Verification items for the finished model (mm, model axes). A direction names the side the tool comes from. Round coordinates to 2 decimals unless told otherwise and drop trailing zeros. Write each loop counter-clockwise with the first axis right and the second up, starting at its lowest first coordinate (ties: lowest second). Pieces come first, ordered by that corner, then holes. Notation, with made-up numbers: M 57,-26 L 76,-26 A23 ccw 76,0 Z; hole C -3.5,-6 d11. An arc over 180 degrees is marked long. One line per item, written item: value. Start each with the question number.
Item 1: Section check A-A, the plane x = -42. Record the cut outline in (y, z), then the cut area to 3 significant figures.
Item 2: Section check B-B, the plane y = -36. Record the cut outline in (x, z), then the cut area to 3 significant figures.
Item 3: Gauge pin test, flat ends, axial feed: pin 1 (14.5 mm diameter, centred on y = 8.5, z = 62.5, fed in from +X); pin 2 (12 mm diameter, centred on y = -6.5, z = 33, fed in from +X); pin 3 (23 mm diameter, centred on x = 38, z = 7.5, fed in from -Y). Record the tip position at first contact, or that the pin passes through.
Item 4: Draft check along X on faces 4 (the face through (-30, 1, 25.4)), 5 (the face through (53.34, 0, 13)), 6 (the face through (-5.74, 28, 13)), 7 (the face through (1.12, -16.22, 12.2)). Enter one of: +X half, -X half, draft (parallel to the pull), parting line (faces both ways), or undercut.
Item 5: Section check C-C, the plane z = 6. Record the cut outline in (x, y).
Item 6: Tool access check on faces 1 (the face through (8.557, 27, 13)), 2 (the face through (1, -22, 24.745)), 3 (the face through (38, -31.519, 13)). Record the directions out of +Z, -Z, +X, -X, +Y, -Y that give a thin tool (end or side, any length) a straight path to the whole face; none if there is none.
Item 7: Thickness scan on probe 1 along Y at (x, z) = (-44, 10); probe 2 along X at (y, z) = (22, 20.5); probe 3 along X at (y, z) = (0, 64). Record the ranges inside material, lowest first. Write a range as from..to.
from build123d import *

# Parameters (mm, degrees)
F1_DEPTH       = 25.4
F2_R           = 5.4495134178
F2_R_2         = 5.5089125438
F3_DEPTH       = 25.4
F4_R           = 5.1025387704
F4_R_2         = 4.874193153
F5_DEPTH       = 25.4
F7_DEPTH       = 25.4
F9_DEPTH       = 25.4
F10_R          = 5.08
F15_R          = 7.7344411216
F16_DEPTH      = 25.4
F17_W          = 15.24
F17_H          = 33.801519665
F18_DEPTH      = 25.4
F18_DEPTH_BACK = 25.4


# Not quite as in the source:
# - a feature of the source that left no trace in its solid (it failed there, or was rolled back) is left out


with BuildPart() as f1:
    # F0 (on Top) → F1 (new body)
    with BuildSketch(Plane.XY):
        with BuildLine():
            Line((-53.3399991691, -31.5190926194), (-27.1817994649, -31.5190926194))
            ThreePointArc((-27.1817994649, -31.5190926194), (-41.6209493128, 0), (-27.1817994649, 31.5190926194))
            Line((-27.1817994649, 31.5190926194), (-53.3399991691, 31.5190926194))
            Line((-53.3399991691, 31.5190926194), (-53.3399991691, -31.5190926194))
        make_face()
        with BuildLine():
            Line((27.1817994649, -31.5190926194), (53.3399991691, -31.5190926194))
            Line((53.3399991691, -31.5190926194), (53.3399991691, 31.5190926194))
            Line((53.3399991691, 31.5190926194), (27.1817994649, 31.5190926194))
            ThreePointArc((27.1817994649, 31.5190926194), (37.8393691772, 17.3345193752), (41.6209493128, 0))
            ThreePointArc((41.6209493128, 0), (37.8393691772, -17.3345193752), (27.1817994649, -31.5190926194))
        make_face()
        with BuildLine():
            ThreePointArc((-27.1817994649, -31.5190926194), (0, -41.6209493128), (27.1817994649, -31.5190926194))
            Line((27.1817994649, -31.5190926194), (-27.1817994649, -31.5190926194))
        make_face()
        with BuildLine():
            Line((-27.1817994649, 31.5190926194), (27.1817994649, 31.5190926194))
            ThreePointArc((27.1817994649, 31.5190926194), (0, 41.6209493128), (-27.1817994649, 31.5190926194))
        make_face()
        with BuildLine():
            Line((-27.1817994649, -31.5190926194), (27.1817994649, -31.5190926194))
            ThreePointArc((27.1817994649, -31.5190926194), (37.8393691772, -17.3345193752), (41.6209493128, 0))
            ThreePointArc((41.6209493128, 0), (37.8393691772, 17.3345193752), (27.1817994649, 31.5190926194))
            Line((27.1817994649, 31.5190926194), (-27.1817994649, 31.5190926194))
            ThreePointArc((-27.1817994649, 31.5190926194), (-41.6209493128, 0), (-27.1817994649, -31.5190926194))
        make_face()
    extrude(amount=F1_DEPTH)

    # F2 (on face) → F3 (cut)
    with BuildSketch(Plane.XY.offset(25.4)):
        with Locations((-44.2123003304, 23.8175932318)):
            Circle(F2_R)
        with Locations((-43.9270585775, -22.6766318083)):
            Circle(F2_R_2)
    extrude(amount=-F3_DEPTH, mode=Mode.SUBTRACT)

    # F4 (on face) → F5 (cut)
    with BuildSketch(Plane.XY.offset(25.4)):
        with Locations((46.7794649303, 24.6733147651)):
            Circle(F4_R)
        with Locations((46.2089851499, -25.2437964082)):
            Circle(F4_R_2)
    extrude(amount=-F5_DEPTH, mode=Mode.SUBTRACT)

    # F6 (on face) → F7 (cut)
    with BuildSketch(Plane.XY.offset(25.4)):
        with BuildLine():
            Line((-6.9852194627, -11.5522462875), (-6.9852194627, -41.0305999317))
            Line((-6.9852194627, -41.0305999317), (6.9852194627, -41.0305999317))
            ThreePointArc((6.9852194627, -41.0305999317), (8.0592339465, -40.8332238489), (9.1277007014, -40.6077394299))
            Line((9.1277007014, -40.6077394299), (9.1277007014, -11.5522462875))
            Line((9.1277007014, -11.5522462875), (-6.9852194627, -11.5522462875))
        make_face()
        with BuildLine():
            Line((6.9852194627, -41.0305999317), (-6.9852194627, -41.0305999317))
            ThreePointArc((-6.9852194627, -41.0305999317), (0, -41.6209493128), (6.9852194627, -41.0305999317))
        make_face()
        with BuildLine():
            Line((5.7398033244, 41.2232710917), (-5.7398033244, 41.2232710917))
            Line((-5.7398033244, 41.2232710917), (-5.7398033244, 11.2670054659))
            Line((-5.7398033244, 11.2670054659), (8.5572190583, 11.2670054659))
            Line((8.5572190583, 11.2670054659), (8.5572190583, 40.7317741289))
            ThreePointArc((8.5572190583, 40.7317741289), (7.1527340625, 41.0017294407), (5.7398033244, 41.2232710917))
        make_face()
    extrude(amount=-F7_DEPTH, mode=Mode.SUBTRACT)

    # F9 (cut): a face of the model
    f9_faces = [f1.faces().sort_by_distance(p)[0] for p in [
        (0, 41.2232710917, 12.7),
    ]]
    extrude(f9_faces, amount=-F9_DEPTH, mode=Mode.SUBTRACT)

    # F10
    f10_edges = [f1.edges().sort_by_distance(p)[0] for p in [
        (53.339999, -31.519093, 12.7),
        (53.339999, 31.519093, 12.7),
        (-53.339999, -31.519093, 12.7),
        (-53.339999, 31.519093, 12.7),
    ]]
    fillet(f10_edges, radius=F10_R)

    # F11 (on Front) → F12 (revolve)
    with BuildSketch(Plane.XZ):
        Polygon((-16.2587165833, 0), (0, 0), (0, 76.0166272521), (-16.2587165833, 76.0166272521), (-16.2587165833, 42.7147820592), (-16.2587165833, 24.7446224093), align=None)
    revolve(axis=Axis((0, 0, 38.0083136261), (0, 0, 1)))

    # F11 (on Front) → F13 (revolve)
    with BuildSketch(Plane.XZ):
        Polygon((-16.2587165833, 0), (0, 0), (0, 76.0166272521), (-16.2587165833, 76.0166272521), (-16.2587165833, 42.7147820592), (-16.2587165833, 24.7446224093), align=None)
        with BuildLine():
            Line((-27.8109610081, 24.7446224093), (-16.2587165833, 24.7446224093))
            Line((-16.2587165833, 24.7446224093), (-16.2587165833, 42.7147820592))
            ThreePointArc((-16.2587165833, 42.7147820592), (-25.501298739, 35.958140564), (-27.8109610081, 24.7446224093))
        make_face()
    revolve(axis=Axis((0, 0, 76.0166272521), (0, 0, -1)))

    # F15 (on face) → F16 (cut)
    with BuildSketch(Plane.XY.offset(76.0166272521)):
        Circle(F15_R)
    extrude(amount=-F16_DEPTH, mode=Mode.SUBTRACT)

    # F17 (on Front) → F18 (cut, two sides)
    with BuildSketch(Plane.XZ) as f18_sk:
        with Locations((0, 69.9550167755)):
            Rectangle(F17_W, F17_H)
    extrude(amount=-F18_DEPTH, mode=Mode.SUBTRACT)
    extrude(f18_sk.sketch, amount=F18_DEPTH_BACK, mode=Mode.SUBTRACT)


solid = f1.part
Response values:
1. outline: M -31.52,0 L -27.84,0 L -27.84,25.4 L -31.52,25.4 Z; M -17.52,0 L 18.84,0 L 18.84,25.4 L -17.52,25.4 Z; M 28.8,0 L 31.52,0 L 31.52,25.4 L 28.8,25.4 Z
1. area: 1,090 mm2
2. outline: M -20.89,0 L -6.99,0 L -6.99,25.4 L -20.89,25.4 Z; M 9.13,0 L 20.89,0 L 20.89,25.4 L 9.13,25.4 Z
2. area: 652 mm2
3. pin 1: stops at x = 16.21
3. pin 2: stops at x = 27.87
3. pin 3: stops at y = -32.09
4. face 4: draft
4. face 5: +X half
4. face 6: undercut
4. face 7: undercut
5. outline: M -53.34,-26.44 A5.08 ccw -48.26,-31.52 L -27.18,-31.52 A41.62 ccw -6.99,-41.03 L -6.99,-14.68 A16.26 ccw 9.13,-13.45 L 9.13,-40.61 A41.62 ccw 27.18,-31.52 L 48.26,-31.52 A5.08 ccw 53.34,-26.44 L 53.34,26.44 A5.08 ccw 48.26,31.52 L 27.18,31.52 A41.62 ccw 8.56,40.73 L 8.56,13.82 A16.26 ccw -5.74,15.21 L -5.74,41.22 A41.62 ccw -27.18,31.52 L -48.26,31.52 A5.08 ccw -53.34,26.44 Z; hole C -44.21,23.82 d10.9; hole C -43.93,-22.68 d11.02; hole C 46.21,-25.24 d9.75; hole C 46.78,24.67 d10.21
6. face 1: -Z, +Y
6. face 2: -Z, -Y
6. face 3: +Z, -Z, +X, -Y
7. probe 1: y = -31.52..-28.19, -17.17..18.37, 29.26..31.52
7. probe 2: x = -53.34..-49.35, -39.07..-5.74, 8.56..42.43, 51.13..53.34
7. probe 3: x = -16.26..-7.73, 7.73..16.26
